Autodesk Inventor part; units mm, degrees
ref_plane "Work Plane1" through (4.3209, 8.636, 0) normal (0, 1, 0) x (1, 0, 0)
ref_plane "YZ Plane" through (0, 0, 0) normal (1, 0, 0) x (0, 1, 0)
ref_plane "XZ Plane" through (0, 0, 0) normal (0, 1, 0) x (-1, 0, 0)
sketch "Sketch2" plane through (0, 0, 0) normal (0, 1, 0) x (-1, 0, 0)
  line L0 (0, 0) -> (23.273, 0)
  line L1 (23.273, 0) -> (23.273, -37.9053)
  line L2 (23.273, -37.9053) -> (0, -37.9053)
  line L3 (0, -37.9053) -> (0, 0)
  line L4 (26.75, 0) -> (-5, 0)
  line L5 (-5, 0) -> (-5, -37.9053)
  line L6 (-5, -37.9053) -> (26.75, -37.9053)
  line L7 (26.75, -37.9053) -> (26.75, 0)
  point P0 (0, -37.9053)
  dimension "d21" = 37.9053
  dimension "d22" = 23.273
  dimension "d36" = 5
  dimension "d37" = 31.75
extrude "Extrusion1" add sketch "Sketch2" along normal blind 8.636
sketch "Sketch6" plane through (-26.75, 0, 0) normal (0, 0, 1) x (1, 0, 0)
  line L0 (31.75, 0) -> (31.75, 8.636)
  line L1 (31.75, 0) -> (31.75, 8.636)
  line L2 (31.75, 0) -> (0, 0)
  line L3 (30.3918, 0) -> (30.3918, 8.636)
  line L4 (31.75, 8.636) -> (0, 8.636)
  line L5 (30.3918, 8.636) -> (55.3918, 8.636) construction
  line L6 (0, 0) -> (0, 8.636)
  line L7 (0, 0) -> (0, 0.5)
  line L8 (30.3918, 8.636) -> (6.505, 0)
  point P0 (26.75, 0)
  dimension "d38" = 1.3582
  dimension "d41" = 0.5
  dimension "d96" = 25.4
  dimension "d97" = 70.123
extrude "Extrusion2" cut sketch "Sketch6" against normal up to surface (37.9053 mm away) contours L8 L2 L6 L4
sketch "Sketch8" plane through (0, 0, 0) normal (0, -1, 0) x (1, 0, 0)
  line L0 (-26.75, -37.9053) -> (-26.75, 0)
  line L1 (-26.75, -10.922) -> (3, -10.922)
  line L2 (3, -10.922) -> (3, -26.9833)
  line L3 (3, -26.9833) -> (-26.75, -26.9833)
  line L4 (-26.75, -26.9833) -> (-26.75, -10.922)
  line L5 (-26.75, 0) -> (5, 0)
  line L6 (5, -37.9053) -> (-26.75, -37.9053)
  line L7 (5, 0) -> (5, -37.9053)
  point P0 (0, 0)
  point P1 (-26.75, -26.9833)
  dimension "d44" = 10.922
  dimension "d45" = 10.922
  dimension "d46" = 2
extrude "Extrusion3" cut sketch "Sketch8" against normal blind 25.4 contours L0 L1 L2 L3
ref_plane "Work Plane1" through (4.3209, 8.636, 0) normal (0, 1, 0) x (1, 0, 0)
sketch "Sketch12" plane through (0, 0, 0) normal (0, -1, 0) x (1, 0, 0)
  line L0 (3.6418, 0) -> (-26.75, 0)
  line L1 (-26.75, 0) -> (0, 0)
  line L2 (0, 0) -> (0, -5)
  line L3 (0, -5) -> (-26.75, -5)
  line L4 (-26.75, -5) -> (-26.75, 0)
  line L5 (-26.75, -37.9053) -> (0, -37.9053)
  line L6 (0, -37.9053) -> (0, -32.9053)
  line L7 (0, -32.9053) -> (-26.75, -32.9053)
  line L8 (-26.75, -32.9053) -> (-26.75, -37.9053)
  line L9 (5, 0) -> (0, 0)
  line L10 (0, 0) -> (0, -1)
  line L11 (0, -1) -> (5, -1)
  line L12 (5, -1) -> (5, 0)
  line L13 (5, 0) -> (5, -37.9053)
  line L14 (5, -37.9053) -> (0, -37.9053)
  line L15 (0, -37.9053) -> (0, -36.9053)
  line L16 (0, -36.9053) -> (5, -36.9053)
  line L17 (5, -36.9053) -> (5, -37.9053)
  line L18 (5, -37.9053) -> (-26.75, -37.9053)
  point P0 (0, -37.9053)
  dimension "d69" = 5
  dimension "d70" = 5
  dimension "d73" = 1
  dimension "d74" = 1
  dimension "d75" = 0
extrude "Extrusion6" cut sketch "Sketch12" along normal through all both and the other way through all
sketch "Sketch13" plane through (0, 0, -36.9053) normal (-1, 0, 0) x (0, 0, 1)
  circle A0 centre (2, 3.9204) radius 1.5
  circle A1 centre (33.9053, 3.9204) radius 1.5
  line L0 (35.9053, 0) -> (31.9053, 0)
  line L1 (31.9053, 7.8408) -> (35.9053, 7.8408)
  line L2 (35.9053, 7.3193) -> (35.9053, 0)
  line L3 (31.9053, 2) -> (31.9053, 7.8408)
  line L4 (0, 0) -> (0, 7.3193)
  line L5 (0, 7.8408) -> (4, 7.8408)
  line L6 (4, 0) -> (0, 0)
  point P0 (36.9053, 0)
  point P1 (35.9053, 8.636)
  point P2 (0, 8.636)
  dimension "d80" = 3
  dimension "d81" = 3
  dimension "d82" = 7.8408
  dimension "d83" = 3.9204
  dimension "d84" = 4
  dimension "d85" = 2
  dimension "d86" = 2
  dimension "d87" = 3.9204
  dimension "d88" = 31.9053
  dimension "d148" = 3.9204
extrude "Extrusion7" cut sketch "Sketch13" against normal blind 25.4
sketch "Sketch15" plane through (3, 8.404, -10.922) normal (-0.34, 0.9404, 0) x (0.9404, 0.34, 0)
  circle A0 centre (-20.2688, -2.4315) radius 1.1146
  circle A1 centre (-7.7296, 18.5871) radius 1.229
  line L0 (-20.2688, -2.4315) -> (-20.2688, 18.5871)
  line L1 (-20.2688, 18.5871) -> (-7.7296, 18.5871)
  line L2 (-7.7296, 18.5871) -> (-7.7296, -2.4315)
  line L3 (-7.7296, -2.4315) -> (-20.2688, -2.4315)
  line L4 (-12.8017, 2.62) -> (-12.8017, 13.4413)
  line L5 (-12.8017, 13.4413) -> (-2.355, 13.4413)
  line L6 (-2.355, 13.4413) -> (-2.355, 2.62)
  line L7 (-2.355, 2.62) -> (-12.8017, 2.62)
  line L8 (-22.0403, -4.4694) -> (-22.0403, 20.5306)
  line L9 (-22.0403, 20.5306) -> (1.9597, 20.5306)
  line L10 (1.9597, 20.5306) -> (1.9597, -4.4694)
  line L11 (1.9597, -4.4694) -> (-22.0403, -4.4694)
  line L12 (-3.19, 21.9833) -> (-24.7175, 21.9833)
  line L13 (-24.7175, -5.922) -> (-3.19, -5.922)
  circle A2 centre (-20.2688, 18.5871) radius 1.1245
  line L14 (0, 16.0613) -> (0, 0)
  line L15 (1.9597, -9.922) -> (1.9597, 25.9833)
  circle A3 centre (-7.7296, -2.4315) radius 1.1245
  point P0 (-5.6786, -10.922)
  dimension "d107" = 21.0186
  dimension "d108" = 12.5392
  dimension "d110" = 25
  dimension "d111" = 24
  dimension "d112" = 4.3148
  dimension "d113" = 9.2386
  dimension "d114" = 7.0893
  dimension "d115" = 7.0893
  dimension "d117" = 1.9436
  dimension "d118" = 2.0378
  dimension "d119" = 1.7714
  dimension "d120" = 9.6893
  dimension "d122" = 1.4526
  dimension "d123" = 1.4526
  dimension "d124" = 2.249
  dimension "d133" = 0
  dimension "d134" = 2.249
hole "Hole3" at (-16.0613, 1.5126, -8.4905) at (-4.2691, 5.7759, -8.4905) at (-4.2691, 5.7759, -29.5091) at (-16.0613, 1.5126, -29.5091) direction (0.34, -0.9404, 0) diameter 2.1211 depth 7.1 tip angle 118 countersink diameter 2.125 countersink angle 90
chamfer "Chamfer3" distance 2 distance2 2 1 edges at (3, 0, -18.9526) measured on face at (4.3333, 0, -21.6295)
equation "\"d83\" = 0.5 * d82"
equation "\"d85\" = 0.5 * d84"
equation "\"d86\" = d85"
equation "\"d87\" = d83"
equation "\"d115\" = d114"
equation "\"d122\" = d123"
properties part number "Camera Angle"
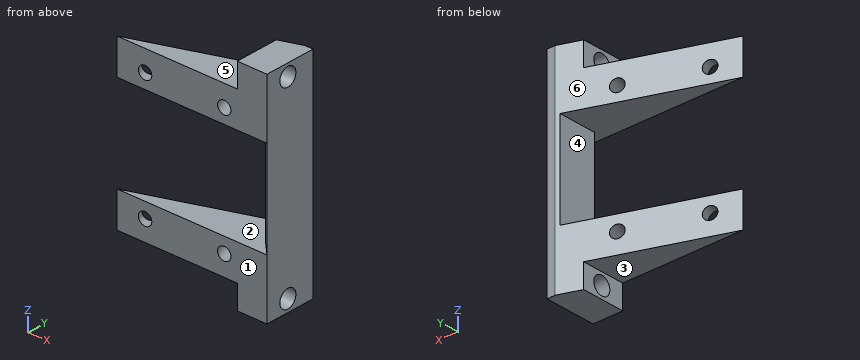
Can you work these out from the model? Positions are in its coordinate system, mm. Face numbers are marked on the shaded views. A direction names the side the tool comes from. Coordinates: 2 decimals unless noted, no trailing zeros. Order: outer loops, then holes, each group sorted by start corner. A loop starts at its lowest first (then second) coordinate and runs counter-clockwise, first axis right, second up. Notation, with made-up numbers: (26.5, 79.5) - (32.5, 79.5) arc R27 cw to (32.5, 114.5) - close; hole circle Ø6 at (78, 75.25). An arc over 180 degrees is marked (long way). Answer as a JSON object with one key per item and string values. Group by question number.
Q1. Imagine slicing it at C-C (x = 1.75). Please give me the cut outline in (y, z), and give its area (3 significant figures).
Q2. Imagine slicing it at A-A (z = -3). Please give me the cut outline in (x, y), and give its area (3 significant figures).
Q3. We'd pull the mould along Z, two halves only. Please class the marked faces 1, 2 and 3: +Z half, -Z half, draft (parallel to the pull), parting line (faces both ways), or undercut.
Q4. I need wall thicknesses on line 1 (Z direction, x = -11.5, y = 2.25); line 2 (Y direction, x = 3.95, z = -3); line 3 (Z direction, x = 2.75, y = 0.75). Which ranges of each line are inside material? Lowest first, please. Write a range as from..to.
Q5. On a 3-axis mill with a long thin cutter (end or side, diameter ignored), from which of +Z, -Z, +X, -X, +Y, -Y can I reach the whole of each face in a straight line? I mean the marked faces 4, 5 and 6. Say none if no direction works.
Q6. Will these pins go through, and if not, where does the flat tip stop? P1, Ø4, axis at y = 4, z = -17.5, coming from the -X side; P2, Ø5, axis at x = -7.5, y = 6.5, coming from the -Z side; P3, Ø3.5, axis at x = -12.5, y = 4.5, coming from the +Z side.
Q7. Imagine slicing it at D-D (y = 4.5). Give the number of separate pieces and of enclosed holes in the cut face, and give its area (3 significant figures).
Q8. Imagine slicing it at B-B (x = -18.25). Please give me the cut outline in (y, z), and give its area (3 significant figures).
Determined:
{
 "1": {"outline": "(0, -36.91) - (7.95, -36.91) - (7.95, -26.98) - (0, -26.98) - close; (0, -10.92) - (7.95, -10.92) - (7.95, -1) - (0, -1) - close; hole circle Ø3 at (3.92, -34.91); hole circle Ø3 at (3.92, -3)", "area": "144 mm2"},
 "2": {"outline": "(0, 0) - (5, 0) - (5, 2.42) - (0, 2.42) - close; (0, 5.42) - (5, 5.42) - (5, 8.64) - (3.64, 8.64) - (0, 7.32) - close", "area": "25.8 mm2"},
 "3": {"face 1": "draft", "face 2": "undercut", "face 3": "-Z half"},
 "4": {"line 1": "z = -32.91..-26.98, -10.92..-5", "line 2": "y = 0..2.42, 5.42..8.64", "line 3": "z = -36.91..-26.98, -10.92..-1"},
 "5": {"face 4": "-X, +Y, -Y", "face 5": "+Z, -X, +Y, -Y", "face 6": "+Z, -Z, -X, +Y"},
 "6": {"P1": "stops at x = 3", "P2": "stops at z = -32.91", "P3": "stops at z = -5"},
 "7": {"separate pieces": "3", "enclosed holes": "2", "area": "189 mm2"},
 "8": {"outline": "(0, -32.91) - (0.72, -32.91) - (0.72, -26.98) - (0, -26.98) - close; (0, -10.92) - (0.72, -10.92) - (0.72, -5) - (0, -5) - close", "area": "8.54 mm2"}
}
